Job drawing, mm, ordinate dimensions from the low corner. One solid piece. A direction names the side the tool comes from. Give positions to 0.01 mm unless a question says otherwise; leave off trailing zeros. Loops run counter-clockwise (first coordinate to the right, second up) from the corner with the lowest first, then second, coordinate; pieces in that order, holes last. Notation, with made-up numbers: (-22, 62) - (22, 62) arc R33 ccw to (22, 93) - close; hole circle Ø9 at (-25.5, 27). An arc over 180 degrees is marked (long way). Answer as CSV lines item,"result". Start each with the question number.
Item 1: Drill centre lines: L1, parallel to X at y = 65.5, z = 37; L2, parallel to Y at x = 23.5, z = 19; L3, parallel to Z at x = 19, y = 61. Where is each one in solid material? Low to high. Write a range as from..to.
Item 2: Saw through at B-B on y = 31. Give the cut face in (x, z).
Item 3: Saw through at A-A on z = 27. Give the cut face in (x, y), plus the area to 3 significant figures.
Item 4: Saw through at C-C on x = 77. Give the cut face in (y, z).
Item 5: Pin check, flat tip, straight feed: pin 1 (1 mm diameter, centred on x = 86, y = 29.5, fed in from +Z). Stop position of the tip, or through.
Item 6: Tool access for the marked faces 1 and 2: list every direction of +Z, -Z, +X, -X, +Y, -Y with a clear straight run to the whole face (end or side of a thin tool).
Item 7: Pull direction X, two halves, no side cores. Call the marked faces 3, 4 and 5: pulls with the +X half, pulls with the -X half, needs draft (parallel to the pull), parting line crosses it, or undercut.
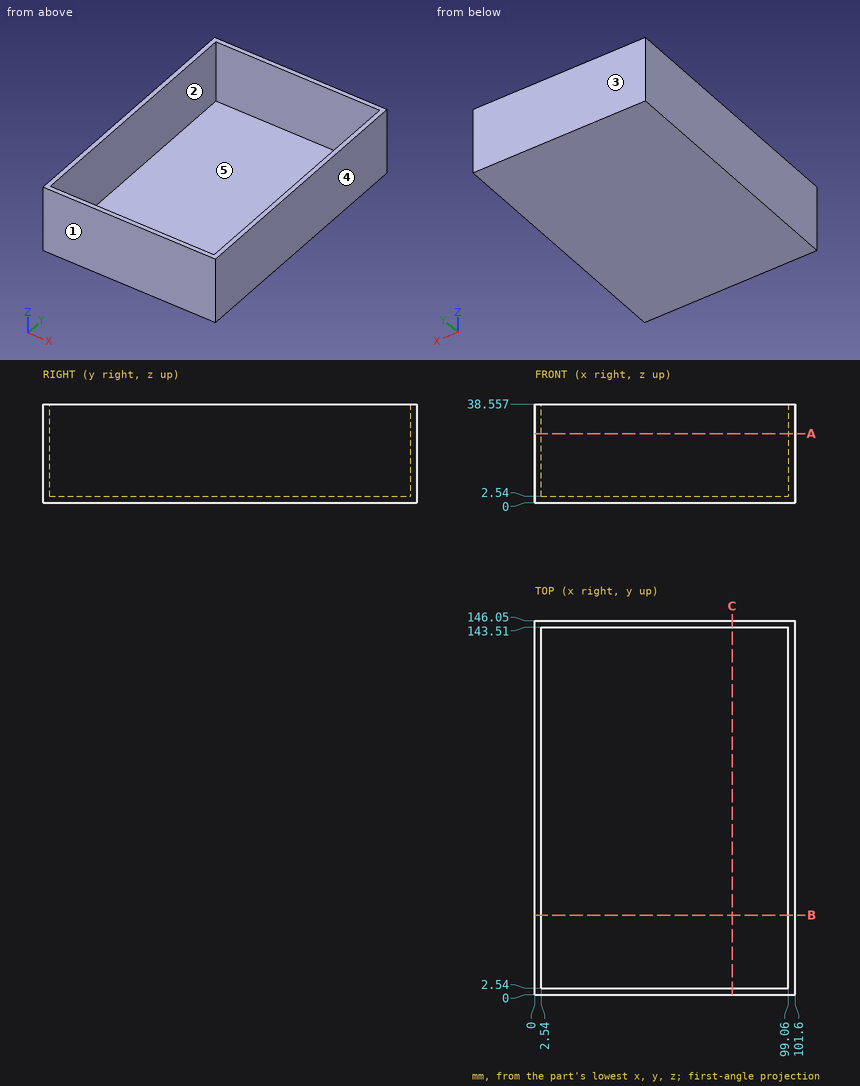
Responses:
1,L1,"0..2.54, 99.06..101.6"
1,L2,"0..2.54, 143.51..146.05"
1,L3,"0..2.54"
2,outline,"(0, 0) - (101.6, 0) - (101.6, 38.56) - (99.06, 38.56) - (99.06, 2.54) - (2.54, 2.54) - (2.54, 38.56) - (0, 38.56) - close"
3,outline,"(0, 0) - (101.6, 0) - (101.6, 146.05) - (0, 146.05) - close; hole (2.54, 2.54) - (99.06, 2.54) - (99.06, 143.51) - (2.54, 143.51) - close"
3,area,"1,230 mm2"
4,outline,"(0, 0) - (146.05, 0) - (146.05, 38.56) - (143.51, 38.56) - (143.51, 2.54) - (2.54, 2.54) - (2.54, 38.56) - (0, 38.56) - close"
5,pin 1,"z = 2.54"
6,face 1,"+Z, -Z, +X, -X, -Y"
6,face 2,"+Z"
7,face 3,"needs draft"
7,face 4,"pulls with the +X half"
7,face 5,"undercut"
